Model file for the job. Use its own axes, mm. Face numbers are marked on the shaded views. A direction names the side the tool comes from. Coordinates: 2 decimals unless noted, no trailing zeros. Write each loop counter-clockwise with the first axis right and the second up, starting at its lowest first coordinate (ties: lowest second). Pieces come first, ordered by that corner, then holes. Notation, with made-up numbers: M 79.5,53 L 91.5,53 A28 cw 91.5,77 Z; hole C 86.25,37 d3. An arc over 180 degrees is marked long. Put each result on its own line as item: value. Start each with the question number.
Q1. Cut at D-D (x = 35). Write the cut outline in (y, z), then the cut area to 3 significant figures.
Q2. Which spindle directions (+Z, -Z, +X, -X, +Y, -Y) get a long thin tool onto all of the face, cutting with end or side? Do the marked faces 1, 2 and 3. Say none if no direction does.
Q3. Cut at A-A (z = 2.75). Write the cut outline in (x, y).
Q4. Cut at B-B (y = 7). Write the cut outline in (x, z).
Q5. Drill centre lines: line 1 along X through (y, z) = (5.75, 2.5); line 2 along Y through (x, z) = (6, 3.15); line 3 along X through (y, z) = (2.5, 7.5). Where is each one in solid material? Low to high.
Q6. Pull direction X, two halves, no side cores. Call the marked faces 4, 5, 6 and 7: pulls with the +X half, pulls with the -X half, needs draft (parallel to the pull), parting line crosses it, or undercut.
Q7. Cut at C-C (z = 10.5). Write the cut outline in (x, y).
Q8. Drop flat-ended pins along their axis: pin 1 (1.5 mm diameter, centred on x = 33.5, y = 2, fed in from +Z); pin 2 (4 mm diameter, centred on x = 27.5, y = 4.5, fed in from +Z); pin 3 (4 mm diameter, centred on x = 7.5, z = 7.5, fed in from +Y); pin 4 (1.7 mm diameter, centred on y = 5.5, z = 6.5, fed in from -X). Give the stop position or say it passes through.
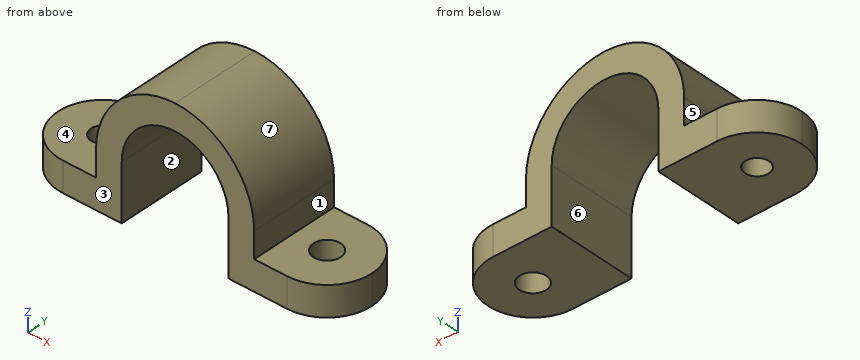
```python
from build123d import *

# Parameters (mm, degrees)
F0_R        = 1.5930303601
F1_DEPTH    = 4
F0_R_2      = 1.8103813353
F0_W        = 18
F0_H        = 12
F0_W_2      = 1.5875
F2_DEPTH    = 18.1281324
F3_R        = 7.14375
F4_DEPTH    = 25.4
F5_W        = 14.2875
F5_H        = 12.0000014
F6_DEPTH    = 7.540625
F7_T1_DEPTH = 65.34


# Not quite as in the source:
# - a fillet or chamfer that OpenCascade refuses, or shapes differently, is made with other operations: its cross-section is extruded or revolved along the edge and cut away or added


with BuildPart() as f1:
    # F0 (on Top) → F1 (new body)
    with BuildSketch(Plane.XY):
        with BuildLine():
            ThreePointArc((0, 6), (1.7573593129, 1.7573593129), (6, 0))
            Line((6, 0), (10.4125, 0))
            Line((10.4125, 0), (10.4125, 12))
            Line((10.4125, 12), (6, 12))
            ThreePointArc((6, 12), (1.7573593129, 10.2426406871), (0, 6))
        make_face()
        with Locations((6, 6)):
            Circle(F0_R, mode=Mode.SUBTRACT)
    extrude(amount=F1_DEPTH)



with BuildPart() as f1b:
    # F0 (on Top) → F1, piece 2 (new body)
    with BuildSketch(Plane.XY):
        with BuildLine():
            Line((31.5875, 12), (31.5875, 0))
            Line((31.5875, 0), (36, 0))
            ThreePointArc((36, 0), (40.2426406871, 1.7573593129), (42, 6))
            ThreePointArc((42, 6), (40.2426406871, 10.2426406871), (36, 12))
            Line((36, 12), (31.5875, 12))
        make_face()
        with Locations((36, 6)):
            Circle(F0_R_2, mode=Mode.SUBTRACT)
    extrude(amount=F1_DEPTH)


with BuildPart() as f1_1:
    add(f1.part)

    add(f1b.part)  # F2 merges F1b
    # F0 (on Top) → F2 (join)
    with BuildSketch(Plane.XY):
        with Locations((21, 6)):
            Rectangle(F0_W, F0_H)
        with Locations((11.20625, 6)):
            Rectangle(F0_W_2, F0_H)
        with Locations((30.79375, 6)):
            Rectangle(F0_W_2, F0_H)
    extrude(amount=F2_DEPTH)

    # F3 (on face) → F4 (cut)
    with BuildSketch(Plane(origin=(0, 12, 0), x_dir=(-1, 0, 0), z_dir=(0, 1, 0))):
        with Locations((-20.9999947, 7.540625)):
            Circle(F3_R)
    extrude(amount=-F4_DEPTH, mode=Mode.SUBTRACT)

    # F5 (on face) → F6 (cut)
    with BuildSketch(Plane.XY):
        with Locations((20.9999947, 6.0000007)):
            Rectangle(F5_W, F5_H)
    extrude(amount=F6_DEPTH, mode=Mode.SUBTRACT)

    # F7: fillet of radius 10.668 on 2 edges, made by hand

    # F7_s2 → F7_t1 (cut)
    with BuildSketch(Plane.XZ.offset(-38.67)):
        with BuildLine():
            ThreePointArc((10.4125, 7.4601324), (13.5370848583, 15.0035475417), (21.0805, 18.1281324))
            Line((21.0805, 18.1281324), (10.4125, 18.1281324))
            Line((10.4125, 18.1281324), (10.4125, 7.4601324))
        make_face()
        with BuildLine():
            ThreePointArc((20.9195, 18.1281324), (28.4629151417, 15.0035475417), (31.5875, 7.4601324))
            Line((31.5875, 7.4601324), (31.5875, 18.1281324))
            Line((31.5875, 18.1281324), (20.9195, 18.1281324))
        make_face()
    extrude(amount=F7_T1_DEPTH, mode=Mode.SUBTRACT)


solid = f1_1.part
```
Computed values:
1. outline: M 0,0 L 4.49,0 L 4.49,4 L 0,4 Z; M 7.51,0 L 12,0 L 12,4 L 7.51,4 Z
1. area: 35.9 mm2
2. face 1: +Z, +X, +Y, -Y
2. face 2: -Z, +Y, -Y
2. face 3: +Z, -Z, +X, -X, -Y
3. outline: M 6,0 L 13.86,0 L 13.86,12 L 6,12 A6 ccw Z; M 28.14,0 L 36,0 A6 ccw 36,12 L 28.14,12 Z; hole C 6,6 d3.19; hole C 36,6 d3.62
4. outline: M 0.08,0 L 4.76,0 L 4.76,4 L 0.08,4 Z; M 7.24,0 L 13.86,0 L 13.86,7.54 A7.14 cw 28.14,7.54 L 28.14,0 L 34.49,0 L 34.49,4 L 31.59,4 L 31.59,7.46 A10.67 ccw 21,18.13 A10.67 ccw 10.41,7.46 L 10.41,4 L 7.24,4 Z; M 37.51,0 L 41.92,0 L 41.92,4 L 37.51,4 Z
5. line 1: 0.01 to 4.43, 7.57 to 13.86, 28.14 to 34.21, 37.79 to 41.99
5. line 2: 0 to 4.41, 7.59 to 12
5. line 3: 10.41 to 13.86, 28.14 to 31.59
6. face 4: needs draft
6. face 5: pulls with the -X half
6. face 6: undercut
6. face 7: pulls with the +X half
7. outline: M 10.85,0 L 14.5,0 L 14.5,12 L 10.85,12 Z; M 27.5,0 L 31.15,0 L 31.15,12 L 27.5,12 Z
8. pin 1: z = 4
8. pin 2: z = 17.09
8. pin 3: through
8. pin 4: x = 10.41
